from build123d import *

# Parameters (mm, degrees)
SKETCH1_R                = 6
BOSS_EXTRUDE1_DEPTH      = 6
BOSS_EXTRUDE2_DEPTH      = 2
M2_CLEARANCE_HOLE1_D     = 2.2
M2_CLEARANCE_HOLE1_DEPTH = 6


with BuildPart() as part:
    # Sketch1 → Boss-Extrude1 (new body)
    with BuildSketch(Plane(origin=(0, 0, 0), x_dir=(0, 0, -1), z_dir=(1, 0, 0))):
        Circle(SKETCH1_R)
    extrude(amount=-BOSS_EXTRUDE1_DEPTH)

    # Sketch2 → Boss-Extrude2 (add)
    with BuildSketch(Plane(origin=(0, 0, 0), x_dir=(0, 0, -1), z_dir=(1, 0, 0))):
        with BuildLine():
            Line((-2.6, 5.407402334), (-2.6, -5.407402334))
            ThreePointArc((-2.6, -5.407402334), (-6, 0), (-2.6, 5.407402334))
        make_face()
        with BuildLine():
            Line((2.6, -5.407402334), (2.6, 5.407402334))
            ThreePointArc((2.6, 5.407402334), (6, 0), (2.6, -5.407402334))
        make_face()
    extrude(amount=BOSS_EXTRUDE2_DEPTH)

    # M2 Clearance Hole1
    with Locations(Plane(origin=(0, 0, 0), x_dir=(0, 0, -1), z_dir=(1, 0, 0))):
        with Locations((0, 0)):
            Hole(M2_CLEARANCE_HOLE1_D / 2, depth=M2_CLEARANCE_HOLE1_DEPTH)


solid = part.part
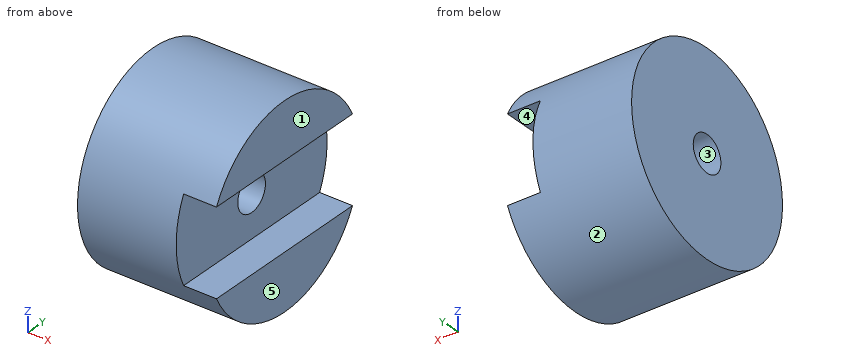
The listing builds one solid part. Answer for the finished solid, in the listing's coordinates (mm). Face numbers are marked on the shaded views. A direction names the side the tool comes from. Give positions to 0.01 mm unless a question says otherwise; leave off trailing zeros. Order: outer loops, then holes, each group sorted by start corner. A loop starts at its lowest first (then second) coordinate and runs counter-clockwise, first axis right, second up. Notation, with made-up numbers: (29.25, 59) - (70.25, 59) arc R20 cw to (70.25, 75) - close; hole circle Ø7 at (-22, 57.25). An arc over 180 degrees is marked (long way). Answer as CSV lines item,"result".
Q1. A cutting plane is placed at B-B, the plane y = 0. Determine the outline of the cut face in (x, z).
Answer key:
outline,"(-6, -6) - (2, -6) - (2, -2.6) - (0, -2.6) - (0, -1.1) - (-6, -1.1) - close; (-6, 1.1) - (0, 1.1) - (0, 2.6) - (2, 2.6) - (2, 6) - (-6, 6) - close"
Q2. Which of the six approach directions +Z, -Z, +X, -X, +Y, -Y give full straight-line access (tool end or side, diameter ignored) to the marked faces 4 and 5?
Answer key:
face 4,"+X, +Y, -Y"
face 5,"+Z, -Z, +X, +Y, -Y"
Q3. Straight lines are drawn through the part: L1, parallel to Y at x = -2.15, z = 0; L2, parallel to Z at x = 0.5, y = -0.25; L3, parallel to X at y = -1.75, z = 0. For each, find the intervals that lie inside material, in ascending order.
Answer key:
L1,"y = -6 to -1.1, 1.1 to 6"
L2,"z = -5.99 to -2.6, 2.6 to 5.99"
L3,"x = -6 to 0"
Q4. A cutting plane is placed at A-A, the plane z = 0. Determine the outline of the cut face in (x, y), and give its area (3 significant figures).
Answer key:
outline,"(-6, -6) - (0, -6) - (0, -1.1) - (-6, -1.1) - close; (-6, 1.1) - (0, 1.1) - (0, 6) - (-6, 6) - close"
area,"58.8 mm^2"
Q5. Determine the mould class of the marked faces 1, 2 and 3 for opening direction Y: pulls with the +Y half, pulls with the -Y half, needs draft (parallel to the pull), parting line crosses it, or undercut.
Answer key:
face 1,"needs draft"
face 2,"parting line crosses it"
face 3,"undercut"
Q6. A cutting plane is placed at D-D, the plane y = 3. Determine the outline of the cut face in (x, z), and give its area (3 significant figures).
Answer key:
outline,"(-6, -5.2) - (2, -5.2) - (2, -2.6) - (0, -2.6) - (0, 2.6) - (2, 2.6) - (2, 5.2) - (-6, 5.2) - close"
area,"72.7 mm^2"
Q7. A cutting plane is placed at C-C, the plane x = -2.5. Determine the outline of the cut face in (y, z), and give its area (3 significant figures).
Answer key:
outline,"circle Ø12 at (0, 0); hole circle Ø2.2 at (0, 0)"
area,"109 mm^2"
Q8. Each of these flat-tipped pins is pushed along its axis until it touches: pin 1 Ø3 at (x, y) = (-0.5, 3.5) entering from +Z; pin 2 Ø1 at (x, y) = (-2, 4) entering from -Z; pin 3 Ø3 at (x, y) = (0.5, 3.5) entering from -Z; pin 4 Ø2 at (y, z) = (0, 0) entering from -X. Where does it stop, or does it pass through?
Answer key:
pin 1,"stops at z = 5.66"
pin 2,"stops at z = -4.87"
pin 3,"stops at z = -5.66"
pin 4,"passes through"
